Verification items for the finished model (mm, model axes). Face numbers are marked on the shaded views. A direction names the side the tool comes from. Coordinates: 2 decimals unless noted, no trailing zeros. Write each loop counter-clockwise with the first axis right and the second up, starting at its lowest first coordinate (ties: lowest second). Pieces come first, ordered by that corner, then holes. Notation, with made-up numbers: (17, -11) -> (35, -11) arc R31 cw to (35, 13) -> close; hole circle Ø6 at (61.5, 25). An arc over 180 degrees is marked (long way). Answer in a Markdown table with one row per item.
```python
from build123d import *

# Parameters (mm, degrees)
SKETCH1_R           = 1.5
BOSS_EXTRUDE1_DEPTH = 3
FILLET1_R           = 2
BOSS_EXTRUDE2_START = 7
SKETCH2_R           = 7.25
BOSS_EXTRUDE2_DEPTH = 6
CHAMFER1_SIZE       = 2
CHAMFER2_SIZE       = 5
CHAMFER3_SIZE       = 1.5


with BuildPart() as part:
    # Sketch1 → Boss-Extrude1 (new body)
    with BuildSketch(Plane.XY):
        Polygon((10, -27.5), (25, -27.5), (25, 27.5), (-5, 27.5), (-5, 20), (-25, 20), (-25, -20), (10, -20), align=None)
        with Locations((0, 22.5)):
            Circle(SKETCH1_R, mode=Mode.SUBTRACT)
        with Locations((20, 22.5)):
            Circle(SKETCH1_R, mode=Mode.SUBTRACT)
        with Locations((20, -22.5)):
            Circle(SKETCH1_R, mode=Mode.SUBTRACT)
    extrude(amount=BOSS_EXTRUDE1_DEPTH)

    # Fillet1
    fillet1_edges = [part.edges().sort_by_distance(p)[0] for p in [
        (25, -27.5, 1.5),
        (-25, -20, 1.5),
        (-25, 20, 1.5),
        (25, 27.5, 1.5),
    ]]
    fillet(fillet1_edges, radius=FILLET1_R)

    # Sketch2 → Boss-Extrude2 (add)
    # profile 1 of 2: a face of its own
    with BuildSketch(Plane(origin=(0, 0, 0), x_dir=(0, 0, -1), z_dir=(1, 0, 0)).offset(BOSS_EXTRUDE2_START)):
        with BuildLine():
            Line((-13, 17), (0, 17))
            Line((0, 17), (0, 29.500000036))
            Line((0, 29.500000036), (-0.98076924, 32.933379086))
            ThreePointArc((-0.98076924, 32.933379086), (-22.979159247, 37.027707534), (-13, 17))
        make_face()
        with Locations((-13, 29.5)):
            Circle(SKETCH2_R, mode=Mode.SUBTRACT)
    # profile 2 of 2: a face of its own
    with BuildSketch(Plane(origin=(0, 0, 0), x_dir=(0, 0, -1), z_dir=(1, 0, 0)).offset(BOSS_EXTRUDE2_START)):
        with BuildLine():
            Line((0, -29.500000036), (-0.98076924, -32.933379086))
            ThreePointArc((-0.98076924, -32.933379086), (-22.979159247, -37.027707534), (-13, -17))
            Line((-13, -17), (0, -17))
            Line((0, -17), (0, -29.500000036))
        make_face()
        with Locations(Location((-13, -29.5, 0), (0, 0, 180))):
            Circle(SKETCH2_R, mode=Mode.SUBTRACT)
    extrude(amount=BOSS_EXTRUDE2_DEPTH)

    # Chamfer1
    chamfer1_edges = [part.edges().sort_by_distance(p)[0] for p in [
        (-5, 20, 1.5),
        (-5, 27.5, 1.5),
    ]]
    chamfer(chamfer1_edges, length=CHAMFER1_SIZE)

    # Chamfer2
    chamfer2_edges = [part.edges().sort_by_distance(p)[0] for p in [
        (10, -17, 3),
        (10, 17, 3),
    ]]
    chamfer(chamfer2_edges, length=CHAMFER2_SIZE)

    # Chamfer3
    chamfer3_edges = [part.edges().sort_by_distance(p)[0] for p in [
        (13, -27.5, 1.5),
        (7, -20, 1.5),
        (13, -19.75, 3),
        (7, -16, 3),
        (7, 27.5, 1.5),
        (13, 27.5, 1.5),
        (7, 19.75, 3),
        (13, 19.75, 3),
    ]]
    chamfer(chamfer3_edges, length=CHAMFER3_SIZE)


solid = part.part
```
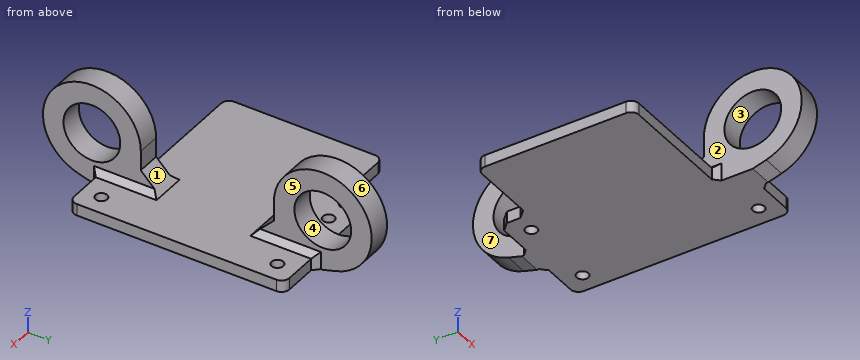
1. Sectioned sample at D-D, the plane x = 11.5. Record the cut outline in (y, z).
Findings below:
| item | result |
|---|---|
| outline | (-32.93, 0.98) -> (-29.5, 0) -> (29.5, 0) -> (32.93, 0.98) arc R12.5 ccw (long way) to (17, 13) -> (17, 8) -> (12, 3) -> (-12, 3) -> (-17, 8) -> (-17, 13) arc R12.5 ccw (long way) to start; hole circle Ø14.5 at (-29.5, 13); hole circle Ø14.5 at (29.5, 13) |
2. Sectioned sample at B-B, the plane z = 22.25. Record the cut outline in (x, y).
Findings below:
| item | result |
|---|---|
| outline | (7, -37.91) -> (13, -37.91) -> (13, -21.09) -> (7, -21.09) -> close; (7, 21.09) -> (13, 21.09) -> (13, 37.91) -> (7, 37.91) -> close |
3. Access from +Z, -Z, +X, -X, +Y, -Y to the whole of each face (thin tool, end or side, straight path). Record for the marked faces 5, 6 and 7.
Findings below:
| item | result |
|---|---|
| face 5 | +Z, +X, +Y |
| face 6 | +X, -X |
| face 7 | +Z, -X, +Y |
4. Go/stop test with flat-tipped pins: pin 1 (6 mm diameter, centred on x = -10, z = 5, fed in from +Y); pin 2 (0.9 mm diameter, centred on x = -6.5, z = 2, fed in from -Y); pin 3 (10 mm diameter, centred on x = 20, y = -17, fed in from +Z); pin 4 (3.5 mm diameter, centred on x = 0, y = 22.5, fed in from -Z). Record where each tip stops, or that it passes through.
Findings below:
| item | result |
|---|---|
| pin 1 | stops at y = 20 |
| pin 2 | stops at y = -20 |
| pin 3 | stops at z = 3 |
| pin 4 | stops at z = 0 |
5. Release check for a two-part mould opening along Z. For the marked faces 1, 2, 3 and 4 record: released by +Z, released by -Z, zero draft, split by the parting line, or undercut.
Findings below:
| item | result |
|---|---|
| face 1 | released by +Z |
| face 2 | zero draft |
| face 3 | undercut |
| face 4 | undercut |
6. Sectioned sample at C-C, the plane y = -14.5. Record the cut outline in (x, z).
Findings below:
| item | result |
|---|---|
| outline | (-25, 0) -> (25, 0) -> (25, 3) -> (14.5, 3) -> (13, 4.5) -> (13, 5.5) -> (7, 5.5) -> (7, 4.5) -> (5.5, 3) -> (-25, 3) -> close |
7. Sectioned sample at A-A, the plane x = 20. Record the cut outline in (y, z), and give its area (3 significant figures).
Findings below:
| item | result |
|---|---|
| outline | (-27.5, 0) -> (-24, 0) -> (-24, 3) -> (-27.5, 3) -> close; (-21, 0) -> (21, 0) -> (21, 3) -> (-21, 3) -> close; (24, 0) -> (27.5, 0) -> (27.5, 3) -> (24, 3) -> close |
| area | 147 mm² |
8. Material ranges on probe 1 along Y at (x, z) = (20, 2.05); probe 2 along Z at (x, y) = (11.2, -29.5); probe 3 along Y at (x, z) = (11.5, 14.25), recorded low to high. Write a range as from..to.
Findings below:
| item | result |
|---|---|
| probe 1 | y = -27.5..-24, -21..21, 24..27.5 |
| probe 2 | z = 0..5.75, 20.25..25.5 |
| probe 3 | y = -41.94..-36.64, -22.36..-17.06, 17.06..22.36, 36.64..41.94 |
